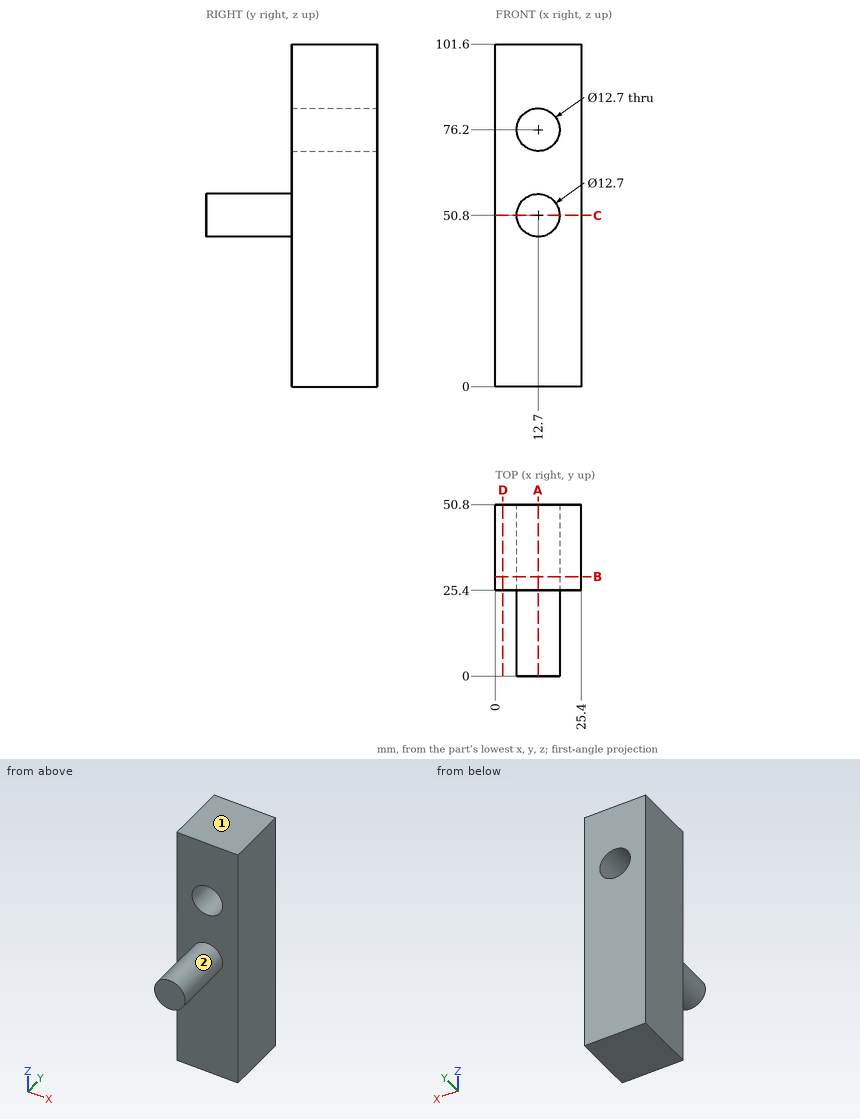
The drawing under review shows one solid part. Ordinate dimensions are in mm from its lowest x, y, z. A direction names the side the tool comes from. Give positions to 0.01 mm unless a question says otherwise; leave off trailing zeros. Order: outer loops, then holes, each group sorted by start corner. A loop starts at its lowest first (then second) coordinate and runs counter-clockwise, first axis right, second up. Notation, with made-up numbers: (77, 85) -> (96, 85) arc R27 cw to (96, 106) -> close; hole circle Ø6 at (28.25, 80.5). An arc over 180 degrees is marked (long way). Write item = value, one per line. Start each with the question number.
(1) For the marked faces 1 and 2, list the 3-axis set-ups (+Z, -Z, +X, -X, +Y, -Y) from which the entire face can be reached by the end or side of a thin tool; tool diameter is ignored.
(2) We need section B-B on y = 29.5. Write out the cut boundary in (x, z), plus the area to 3 significant figures.
(3) To check wall thickness, follow line 1 along Z through (x, y) = (12.7, 33.5); line 2 along X through (y, z) = (44, 76.2); line 3 along Y through (x, z) = (24.25, 68). State the ranges of each line that lie inside material, in increasing order.
(4) We need section A-A on x = 12.7. Write out the cut boundary in (y, z), plus the area to 3 significant figures.
(5) We need section C-C on z = 50.8. Write out the cut boundary in (x, y), plus the area to 3 significant figures.
(6) We need section D-D on x = 2.25. Write out the cut boundary in (y, z), plus the area to 3 significant figures.
(7) For pin 1 (12 mm diameter, centred on x = 21.5, z = 31.5, fed in from -Y); pin 2 (7.5 mm diameter, centred on x = 14.5, z = 52, fed in from -Y); pin 3 (10 mm diameter, centred on x = 12.7, z = 76.2, fed in from +Y), all flat-tipped, find the tip position at first contact; note any pin that passes through.
Numbers:
q1.face_1 = +Z, +X, -X, +Y, -Y
q1.face_2 = -Y
q2.outline = (0, 0) -> (25.4, 0) -> (25.4, 101.6) -> (0, 101.6) -> close; hole circle Ø12.7 at (12.7, 76.2)
q2.area = 2,450 mm^2
q3.line_1 = 0 to 69.85, 82.55 to 101.6
q3.line_2 = 0 to 6.35, 19.05 to 25.4
q3.line_3 = 25.4 to 50.8
q4.outline = (0, 44.45) -> (25.4, 44.45) -> (25.4, 0) -> (50.8, 0) -> (50.8, 69.85) -> (25.4, 69.85) -> (25.4, 57.15) -> (0, 57.15) -> close; (25.4, 82.55) -> (50.8, 82.55) -> (50.8, 101.6) -> (25.4, 101.6) -> close
q4.area = 2,580 mm^2
q5.outline = (0, 25.4) -> (6.35, 25.4) -> (6.35, 0) -> (19.05, 0) -> (19.05, 25.4) -> (25.4, 25.4) -> (25.4, 50.8) -> (0, 50.8) -> close
q5.area = 968 mm^2
q6.outline = (25.4, 0) -> (50.8, 0) -> (50.8, 101.6) -> (25.4, 101.6) -> close
q6.area = 2,580 mm^2
q7.pin_1 = 25.4
q7.pin_2 = 0
q7.pin_3 = through
